Check sheet for the modelled part. Datum: model origin and axes. Units: mm. Face numbers are marked on the shaded views. A direction names the side the tool comes from. Give positions to 0.01 mm unless a question says otherwise; leave off trailing zeros. Loops run counter-clockwise (first coordinate to the right, second up) from the corner with the lowest first, then second, coordinate; pieces in that order, holes last. Notation, with made-up numbers: (36.25, -30.5) - (82.25, -30.5) arc R29 ccw to (82.25, -4.5) - close; hole circle Ø5 at (83, 48). An arc over 180 degrees is marked (long way). Use CSV: the item, a comma, the result in double quotes.
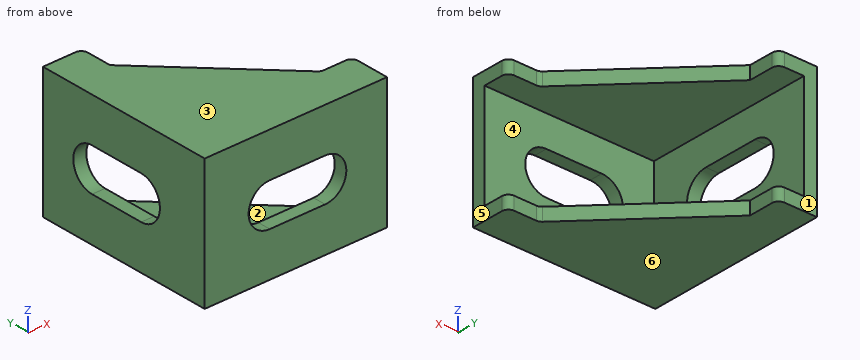
from build123d import *

# Parameters (mm, degrees)
EXTRUDE_1_DEPTH     = 20
SKETCH_2_W          = 16
SKETCH_2_H          = 26
CUT_EXTRUDE_1_DEPTH = 26
CUT_EXTRUDE_2_REACH = 4
CUT_EXTRUDE_3_REACH = 4
FILLET_1_R          = 1


with BuildPart() as part:
    # 草图1 → 凸台-拉伸1 (new body)
    with BuildSketch(Plane.XY):
        Polygon((0, 0), (0, 28), (6, 28), (6, 23.169014085), (23.169014085, 6), (28, 6), (28, 0), align=None)
    extrude(amount=EXTRUDE_1_DEPTH)

    # 草图2 → 切除-拉伸1 (cut)
    with BuildSketch(Plane(origin=(28, 0, 0), x_dir=(0, 0, -1), z_dir=(1, 0, 0))):
        with Locations((-10, 15)):
            Rectangle(SKETCH_2_W, SKETCH_2_H)
    extrude(amount=-CUT_EXTRUDE_1_DEPTH, mode=Mode.SUBTRACT)

    # 草图3 → 切除-拉伸2 (cut, up to next)
    with BuildSketch(Plane(origin=(2, 0, 0), x_dir=(0, 0, -1), z_dir=(1, 0, 0)), mode=Mode.PRIVATE) as cut_extrude_2_sk1:
        with BuildLine():
            Line((-13.25, 11), (-13.25, 19.5))
            ThreePointArc((-13.25, 19.5), (-10, 22.75), (-6.75, 19.5))
            Line((-6.75, 19.5), (-6.75, 11))
            ThreePointArc((-6.75, 11), (-10, 7.75), (-13.25, 11))
        make_face()
    cut_extrude_2_tool1 = extrude(cut_extrude_2_sk1.sketch, amount=-CUT_EXTRUDE_2_REACH, mode=Mode.PRIVATE) & part.part
    add(cut_extrude_2_tool1.solids().sort_by_distance((2, 15.25, 10))[0], mode=Mode.SUBTRACT)

    # 草图4 → 切除-拉伸3 (cut, up to next)
    with BuildSketch(Plane(origin=(0, 2, 2), x_dir=(1, 0, 0), z_dir=(0, 1, 0)), mode=Mode.PRIVATE) as cut_extrude_3_sk1:
        with BuildLine():
            Line((10, -4.75), (18.5, -4.75))
            ThreePointArc((18.5, -4.75), (21.75, -8), (18.5, -11.25))
            Line((18.5, -11.25), (10, -11.25))
            ThreePointArc((10, -11.25), (6.75, -8), (10, -4.75))
        make_face()
    cut_extrude_3_tool1 = extrude(cut_extrude_3_sk1.sketch, amount=-CUT_EXTRUDE_3_REACH, mode=Mode.PRIVATE) & part.part
    add(cut_extrude_3_tool1.solids().sort_by_distance((14.25, 2, 10))[0], mode=Mode.SUBTRACT)

    # 圆角1
    fillet_1_edges = [part.edges().sort_by_distance(p)[0] for p in [
        (6, 28, 19),
        (23.169014085, 6, 19),
        (28, 6, 19),
        (6, 28, 1),
        (23.169014085, 6, 1),
        (28, 6, 1),
    ]]
    fillet(fillet_1_edges, radius=FILLET_1_R)


solid = part.part
1. Sectioned sample at B-B, the plane y = 17.5. Record the boundary of the cut face in (x, z), and give its area (3 significant figures).
Completed:
outline,"(0, 0) - (11.67, 0) - (11.67, 2) - (2, 2) - (2, 6.75) - (0, 6.75) - close; (0, 13.25) - (2, 13.25) - (2, 18) - (11.67, 18) - (11.67, 20) - (0, 20) - close"
area,"65.7 mm²"
2. Release check for a two-part mould opening along Z. For the marked faces 3, 4, 5 and 6 record: released by +Z, released by -Z, zero draft, split by the parting line, or undercut.
Completed:
face 3,"released by +Z"
face 4,"undercut"
face 5,"zero draft"
face 6,"released by -Z"
3. Sectioned sample at D-D, the plane x = 24.25. Record the boundary of the cut face in (y, z).
Completed:
outline,"(0, 0) - (6, 0) - (6, 2) - (2, 2) - (2, 18) - (6, 18) - (6, 20) - (0, 20) - close"
4. Set-up check for the marked faces 1 and 2: record each of +Z, -Z, +X, -X, +Y, -Y from which the full face is reachable in a straight line by a thin tool's end or side.
Completed:
face 1,"+Z, -Z, +X, -X, +Y"
face 2,"+X, +Y"
5. Sectioned sample at C-C, the plane y = 3.25. Record the boundary of the cut face in (x, z).
Completed:
outline,"(0, 0) - (28, 0) - (28, 2) - (2, 2) - (2, 18) - (28, 18) - (28, 20) - (0, 20) - close"
6. Go/stop test with flat-tipped pins: pin 1 Ø2 at (x, z) = (25.5, 19.5) entering from +Y; pin 2 Ø5 at (y, z) = (20.5, 11.5) entering from +X; pin 3 Ø5 at (y, z) = (10, 2.5) entering from +X. Record where each tip stops, or that it passes through.
Completed:
pin 1,"stops at y = 6"
pin 2,"stops at x = 2"
pin 3,"stops at x = 21.62"
7. Scan lines: line 1 along Z through (x, y) = (7, 17); line 2 along Y through (x, z) = (8, 4.75). Record each from-to range of solid material in increasing order.
Completed:
line 1,"z = 0 to 2, 18 to 20"
line 2,"y = 0 to 2"
8. Sectioned sample at A-A, the plane z = 10. Record the boundary of the cut face in (x, y), and give its area (3 significant figures).
Completed:
outline,"(0, 0) - (6.75, 0) - (6.75, 2) - (2, 2) - (2, 7.75) - (0, 7.75) - close; (0, 22.75) - (2, 22.75) - (2, 28) - (0, 28) - close; (21.75, 0) - (28, 0) - (28, 2) - (21.75, 2) - close"
area,"48.0 mm²"
